Autodesk Fusion 360 part; units mm, degrees
sketch "Sketch1" plane through (0, 0, 0) normal (0, 0, 1) x (1, 0, 0)
  line L0 (10, -2.5) -> (10, -4)
  line L1 (10, -4) -> (4, -4)
  line L2 (4, -4) -> (4, -6.6)
  line L3 (4, -6.6) -> (6, -6.6)
  line L4 (6, -6.6) -> (6, -9.1)
  line L5 (6, -9.1) -> (2.5, -9.1)
  line L6 (2.5, -9.1) -> (2.5, -4.0389)
  line L7 (-2.5, -4.0389) -> (-2.5, -9.1)
  line L8 (-2.5, -9.1) -> (-6, -9.1)
  line L9 (-6, -9.1) -> (-6, -6.6)
  line L10 (-6, -6.6) -> (-4, -6.6)
  line L11 (-4, -6.6) -> (-4, -4)
  line L12 (-4, -4) -> (-10, -4)
  line L13 (-10, -4) -> (-10, -2.5)
  line L14 (-10, -2.5) -> (-5.75, -2.5)
  line L15 (5.75, -2.5) -> (10, -2.5)
  arc A0 (2.5, -4.0389) -> (-2.5, -4.0389) centre (0, 0) ccw
  arc A1 (5.75, 0) -> (-5.75, 0) centre (0, 0) ccw
  line L16 (-5.75, 0) -> (-5.75, -2.5)
  line L17 (5.75, 0) -> (5.75, -2.5)
  dimension "d3" = 8
  dimension "d4" = 4
  dimension "d5" = 5
  dimension "d6" = 2.5
  dimension "d7" = 2.5
  dimension "d8" = 2.6
  dimension "d9" = 12
  dimension "d10" = 20
  dimension "d11" = 6
  dimension "d12" = 10
  dimension "d14" = 2.5
  dimension "d19" = 9.5
  dimension "d24" = 1.5
  dimension "d25" = 11.5
extrude "Extrude1" add sketch "Sketch1" along normal blind 10
chamfer "Chamfer1" distance 0.75 angle 45 4 edges at (-6, -6.6, 5) (-6, -9.1, 5) (6, -6.6, 5) (6, -9.1, 5)
fillet "Fillet3" radius 2 2 edges at (-5.75, -2.5, 5) (5.75, -2.5, 5)
equation "d4 = d3 / 2"
equation "d6 = d5 / 2"
equation "d11 = d9 / 2"
equation "d12 = d10 / 2"
Build history of the part. All positions in model axes, mm. A direction names the side the tool comes from. Give positions to 0.01 mm unless a question says otherwise; leave off trailing zeros. Write each loop counter-clockwise with the first axis right and the second up, starting at its lowest first coordinate (ties: lowest second). Pieces come first, ordered by that corner, then holes. Notation, with made-up numbers: (40, -37.5) - (44, -37.5) arc R24 ccw to (44, -4.5) - close; hole circle Ø3 at (75, 78.5). An arc over 180 degrees is marked (long way). Use one line per item in the form item = value. Start each with the question number.
1. 3-axis set-ups, long thin cutter, end or side, ignore diameter. For faces 4 (the face through (-9, -2.5, 5)), 5 (the face through (9, -2.5, 5)), 6 (the face through (-2.5, -7, 5)), 7 (the face through (-4, -5, 5)): which of +Z, -Z, +X, -X, +Y, -Y reach the whole face in a straight line?
2. Band-saw the part on D-D on x = 0. Write the cut outline in (y, z).
3. Band-saw the part on C-C on x = -3. Write the cut outline in (y, z).
4. Two-plate mould, pull along Y, no slides. Class faces 1 (the face through (4, -5, 5)), 2 (the face through (6.32, -1.9, 5.07)), 3 (the face through (-10, -3, 5)): released by +Y, released by -Y, zero draft, split by the parting line, or undercut.
5. Probe line 1 (X direction, y = 0, z = 7); line 2 (X direction, y = -5, z = 9); line 3 (Y direction, x = 0, z = 7). List the from-to ranges inside material, lowest first. Write a range as [from, to].
6. Drop flat-ended pins along their axis: pin 1 Ø5.5 at (y, z) = (-7.5, 4.5) entering from +X; pin 2 Ø0.6 at (x, z) = (-5, 3) entering from +Y; pin 3 Ø5 at (x, z) = (7.5, 3.5) entering from -Y; pin 4 Ø1.8 at (x, z) = (-8.5, 5) entering from +Y. Give the stop position or say it passes through.
7. Band-saw the part on A-A on y = -8. Write the cut outline in (x, z).
8. Band-saw the part on B-B on z = 4.25. Write the cut outline in (x, y).
Conclusion:
q1.face_4 = +Z, -Z, -X, +Y
q1.face_5 = +Z, -Z, +X, +Y
q1.face_6 = +Z, -Z, -Y
q1.face_7 = +Z, -Z, -X
q2.outline = (4.75, 0) - (5.75, 0) - (5.75, 10) - (4.75, 10) - close
q3.outline = (-9.1, 0) - (-3.68, 0) - (-3.68, 10) - (-9.1, 10) - close; (3.68, 0) - (4.91, 0) - (4.91, 10) - (3.68, 10) - close
q4.face_1 = undercut
q4.face_2 = released by +Y
q4.face_3 = zero draft
q5.line_1 = [-5.75, -4.75], [4.75, 5.75]
q5.line_2 = [-4, -2.5], [2.5, 4]
q5.line_3 = [4.75, 5.75]
q6.pin_1 = 6
q6.pin_2 = 3.31
q6.pin_3 = -9.1
q6.pin_4 = -2.49
q7.outline = (-6, 0) - (-2.5, 0) - (-2.5, 10) - (-6, 10) - close; (2.5, 0) - (6, 0) - (6, 10) - (2.5, 10) - close
q8.outline = (-10, -4) - (-4, -4) - (-4, -6.6) - (-5.25, -6.6) - (-6, -7.35) - (-6, -8.35) - (-5.25, -9.1) - (-2.5, -9.1) - (-2.5, -4.04) arc R4.75 cw (long way) to (2.5, -4.04) - (2.5, -9.1) - (5.25, -9.1) - (6, -8.35) - (6, -7.35) - (5.25, -6.6) - (4, -6.6) - (4, -4) - (10, -4) - (10, -2.5) - (7.75, -2.5) arc R2 cw to (5.75, -0.5) - (5.75, 0) arc R5.75 ccw to (-5.75, 0) - (-5.75, -0.5) arc R2 cw to (-7.75, -2.5) - (-10, -2.5) - close
